Autodesk Inventor part; units mm, degrees
ref_plane "YZ Plane" through (0, 0, 0) normal (1, 0, 0) x (0, 1, 0)
ref_plane "XZ Plane" through (0, 0, 0) normal (0, 1, 0) x (-1, 0, 0)
ref_plane "XY Plane" through (0, 0, 0) normal (0, 0, 1) x (1, 0, 0)
sketch "Sketch1" plane through (0, 0, 0) normal (0, 0, 1) x (1, 0, 0)
  line L0 (-12.7, -19.05) -> (12.7, -19.05)
  line L1 (12.7, -19.05) -> (12.7, 19.05)
  line L2 (12.7, 19.05) -> (-12.7, 19.05)
  line L3 (-12.7, 19.05) -> (-12.7, -19.05)
  line L4 (-12.7, -19.05) -> (12.7, 19.05) construction
  line L5 (12.7, -19.05) -> (-12.7, 19.05) construction
  line L6 (-9.525, -15.875) -> (9.525, -15.875)
  line L7 (9.525, -15.875) -> (9.525, 15.875)
  line L8 (9.525, 15.875) -> (-9.525, 15.875)
  line L9 (-9.525, 15.875) -> (-9.525, -15.875)
  line L10 (-9.525, -15.875) -> (9.525, 15.875) construction
  line L11 (9.525, -15.875) -> (-9.525, 15.875) construction
  point P0 (0, 0)
  dimension "d0" = 25.4
  dimension "d1" = 38.1
  dimension "d2" = 3.175
  dimension "d3" = 3.175
extrude "Extrusion1" add sketch "Sketch1" along normal mid plane 304.8
sketch "Sketch2" plane through (-12.7, -19.05, 152.4) normal (0, -1, 0) x (1, 0, 0)
  line L0 (25.4, -304.8) -> (0, -304.8)
  line L1 (25.4, -304.8) -> (0, -290.1353)
  line L2 (0, 0) -> (0, -304.8)
  line L3 (0, -304.8) -> (0, -290.1353)
  line L4 (0, -304.8) -> (25.4, -304.8)
  line L5 (22.225, -304.8) -> (22.225, 0)
  point P0 (12.7, -152.4)
  dimension "d6" = 30
extrude "Extrusion2" cut sketch "Sketch2" against normal through all
properties part number "spacerForTopSideAluminumExtrusion" material "Aluminum 6061, Welded"
Read the model definition and answer for the solid it produces. Units are mm, in the model's axes. A direction names the side the tool comes from. Round coordinates to 2 decimals unless told otherwise and drop trailing zeros. Write each loop counter-clockwise with the first axis right and the second up, starting at its lowest first coordinate (ties: lowest second). Pieces come first, ordered by that corner, then holes. Notation, with made-up numbers: (83, 9.25) -> (111, 9.25) arc R17 ccw to (111, 28.25) -> close; hole circle Ø6 at (83, 59.25). An arc over 180 degrees is marked (long way). Answer in a Markdown table with one row per item. Add a question column.
1) Given P1, Ø4, axis at x = 10, y = -8.5, coming from the -Z side, flat-ended and moving along its own axis, determine where the tip first touches the part or whether it passes through.
2) Find section A-A, the plane y = -5. Determine the outline of the cut face in (x, z) (3 decimals).
3) Find section C-C, the plane x = -3. Determine the outline of the cut face in (y, z) (3 decimals).
4) Determine the mould class of faces 1 (the face through (12.7, 0, -2)), 2 (the face through (-9.525, 0, 4)), 3 (the face through (11, 0, 152.4)), 4 (the face through (0, -15.875, -1)) for opening direction X: pulls with the +X half, pulls with the -X half, needs draft (parallel to the pull), parting line crosses it, or undercut.
5) Find section B-B, the plane z = 116. Determine the outline of the cut face in (x, y) (3 decimals).
6) Consider line 1 (X direction, y = 0.5, z = 130) (3 decimals); line 2 (Y direction, x = -4, z = 3) (3 decimals); line 3 (Z direction, x = 10.25, y = -13). Determine where each line is inside the solid, lowest interval first.
7) Which of the six approach directions +Z, -Z, +X, -X, +Y, -Y give full straight-line access (tool end or side, diameter ignored) to faces 5 (the face through (0, -19.05, -2)), 6 (the face through (0, 15.875, -1))?
Findings below:
| question | item | result |
|---|---|---|
| 1 | P1 | z = -152 |
| 2 | outline | (-12.7, -137.735) -> (-9.525, -139.568) -> (-9.525, 152.4) -> (-12.7, 152.4) -> close; (9.525, -150.567) -> (12.7, -152.4) -> (12.7, 152.4) -> (9.525, 152.4) -> close |
| 3 | outline | (-19.05, -143.336) -> (-15.875, -143.336) -> (-15.875, 152.4) -> (-19.05, 152.4) -> close; (15.875, -143.336) -> (19.05, -143.336) -> (19.05, 152.4) -> (15.875, 152.4) -> close |
| 4 | face 1 | pulls with the +X half |
| 4 | face 2 | undercut |
| 4 | face 3 | needs draft |
| 4 | face 4 | undercut |
| 5 | outline | (-12.7, -19.05) -> (12.7, -19.05) -> (12.7, 19.05) -> (-12.7, 19.05) -> close; hole (-9.525, -15.875) -> (9.525, -15.875) -> (9.525, 15.875) -> (-9.525, 15.875) -> close |
| 6 | line 1 | -12.7 to -9.525, 9.525 to 12.7 |
| 6 | line 2 | -19.05 to -15.875, 15.875 to 19.05 |
| 6 | line 3 | -150.99 to 152.4 |
| 7 | face 5 | +Z, -Z, +X, -X, -Y |
| 7 | face 6 | +Z, -Z |
